Read the model definition and answer for the solid it produces. Units are mm, in the model's axes. A direction names the side the tool comes from. Coordinates: 2 decimals unless noted, no trailing zeros. Order: outer loops, then holes, each group sorted by start corner. A loop starts at its lowest first (then second) coordinate and runs counter-clockwise, first axis right, second up. Notation, with made-up numbers: M 50.5,48 L 100.5,48 A14 cw 100.5,62 Z; hole C 67,-16 d1. An arc over 180 degrees is marked long. Use a Markdown table: item, result. Add a question column.
1) The mould has two halves that part along X. Classify faces 1 (the face through (10, -50.8, 10)), 2 (the face through (130.168, -41, -22)), 3 (the face through (-87.57, -41.41, -3.07)), 4 (the face through (-144.733, -1, -2)): released by +X, released by -X, zero draft, split by the parting line, or undercut.
2) Find section C-C on z = -2. Write down the section's boundary in (x, y), plus the area to 3 significant figures.
3) Find section D-D on y = -36.5. Write down the section's boundary in (x, z) (3 decimals).
4) Each of these flat-tipped pins is pushed along its axis until it touches: pin 1 Ø8 at (y, z) = (-35.5, 50.5) entering from +X; pin 2 Ø7 at (x, y) = (104.5, -45.5) entering from -Z; pin 3 Ø12 at (x, y) = (-70, -25) entering from +Z. Where does it stop, or does it pass through?
5) Find section B-B on x = 44. Write down the section's boundary in (y, z), plus the area to 3 significant figures.
6) Find the intervals of material crossed by probe 1 along Z at (x, y) = (75, 28); probe 2 along Y at (x, z) = (-126.5, -5); probe 3 along X at (y, z) = (-43.5, 20.5), in increasing order. Write a range as [from, to].
7) Find section A-A on y = 30.5. Write down the section's boundary in (x, z).
8) For faces 5 (the face through (-5, -1, 63.942)), 6 (the face through (-107, -41, 3.617)), 7 (the face through (28.568, -1, 41)), 8 (the face through (-104, -1, 25.842)), determine the directions among +Z, -Z, +X, -X, +Y, -Y from which every point of the face is accessible in a straight line to the end or side of a thin tool.
from build123d import *

# Parameters (mm, degrees)
F1_DEPTH = 50.8
F3_DEPTH = 19.05


with BuildPart() as f1:
    # F0 (on Front) → F1 (new body, symmetric)
    with BuildSketch(Plane.XZ):
        with BuildLine():
            Line((-71.399881, 25.841707), (-138.383388, 25.841707))
            ThreePointArc((-138.383388, 25.841707), (-142.873516, 23.981835), (-144.733388, 19.491707))
            Line((-144.733388, 19.491707), (-144.733388, -24.958293))
            Line((-144.733388, -24.958293), (-119.333388, -24.958293))
            Line((-119.333388, -24.958293), (-119.333388, -18.608293))
            ThreePointArc((-119.333388, -18.608293), (-112.823836, -2.892845), (-97.108388, 3.616707))
            Line((-97.108388, 3.616707), (-90.758388, 3.616707))
            ThreePointArc((-90.758388, 3.616707), (-75.042939, -2.892845), (-68.533388, -18.608293))
            Line((-68.533388, -18.608293), (-68.533388, -24.958293))
            Line((-68.533388, -24.958293), (83.866612, -24.958293))
            Line((83.866612, -24.958293), (83.866612, -18.608293))
            ThreePointArc((83.866612, -18.608293), (90.376164, -2.892845), (106.091612, 3.616707))
            Line((106.091612, 3.616707), (112.441612, 3.616707))
            ThreePointArc((112.441612, 3.616707), (128.157061, -2.892845), (134.666612, -18.608293))
            Line((134.666612, -18.608293), (134.666612, -24.958293))
            Line((134.666612, -24.958293), (168.267654, -24.958293))
            Line((168.267654, -24.958293), (168.267654, 25.841707))
            Line((168.267654, 25.841707), (28.567654, 25.841707))
            Line((28.567654, 25.841707), (28.567654, 57.591707))
            ThreePointArc((28.567654, 57.591707), (26.707782, 62.081835), (22.217654, 63.941707))
            Line((22.217654, 63.941707), (-32.065853, 63.941707))
            ThreePointArc((-32.065853, 63.941707), (-34.678483, 63.379337), (-36.828353, 61.791837))
            Line((-36.828353, 61.791837), (-66.637381, 27.991577))
            ThreePointArc((-66.637381, 27.991577), (-68.78725, 26.404077), (-71.399881, 25.841707))
        make_face()
        with BuildLine():
            Line((-119.333388, -18.608293), (-119.333388, -24.958293))
            Line((-119.333388, -24.958293), (-68.533388, -24.958293))
            Line((-68.533388, -24.958293), (-68.533388, -18.608293))
            ThreePointArc((-68.533388, -18.608293), (-75.042939, -2.892845), (-90.758388, 3.616707))
            Line((-90.758388, 3.616707), (-97.108388, 3.616707))
            ThreePointArc((-97.108388, 3.616707), (-112.823836, -2.892845), (-119.333388, -18.608293))
        make_face()
        with BuildLine():
            Line((83.866612, -18.608293), (83.866612, -24.958293))
            Line((83.866612, -24.958293), (134.666612, -24.958293))
            Line((134.666612, -24.958293), (134.666612, -18.608293))
            ThreePointArc((134.666612, -18.608293), (128.157061, -2.892845), (112.441612, 3.616707))
            Line((112.441612, 3.616707), (106.091612, 3.616707))
            ThreePointArc((106.091612, 3.616707), (90.376164, -2.892845), (83.866612, -18.608293))
        make_face()
    extrude(amount=F1_DEPTH, both=True)

    # F2 (on face) → F3 (cut)
    with BuildSketch(Plane.XZ.offset(50.8)):
        with BuildLine():
            Line((-132.033388, -18.608293), (-132.033388, -24.958293))
            Line((-132.033388, -24.958293), (-81.233388, -24.958293))
            Line((-81.233388, -24.958293), (-81.233388, -18.608293))
            ThreePointArc((-81.233388, -18.608293), (-87.742939, -2.892845), (-103.458388, 3.616707))
            Line((-103.458388, 3.616707), (-109.808388, 3.616707))
            ThreePointArc((-109.808388, 3.616707), (-125.523836, -2.892845), (-132.033388, -18.608293))
        make_face()
        with BuildLine():
            Line((79.367654, -18.608293), (79.367654, -24.958293))
            Line((79.367654, -24.958293), (130.167654, -24.958293))
            Line((130.167654, -24.958293), (130.167654, -18.608293))
            ThreePointArc((130.167654, -18.608293), (123.658102, -2.892845), (107.942654, 3.616707))
            Line((107.942654, 3.616707), (101.592654, 3.616707))
            ThreePointArc((101.592654, 3.616707), (85.877206, -2.892845), (79.367654, -18.608293))
        make_face()
    extrude(amount=-F3_DEPTH, mode=Mode.SUBTRACT)


solid = f1.part
Check result:
| question | item | result |
|---|---|---|
| 1 | face 1 | zero draft |
| 1 | face 2 | undercut |
| 1 | face 3 | undercut |
| 1 | face 4 | released by -X |
| 2 | outline | M -144.73,-50.8 L -124.58,-50.8 L -124.58,-31.75 L -88.69,-31.75 L -88.69,-50.8 L 86.82,-50.8 L 86.82,-31.75 L 122.71,-31.75 L 122.71,-50.8 L 168.27,-50.8 L 168.27,50.8 L -144.73,50.8 Z |
| 2 | area | 30,400 mm2 |
| 3 | outline | M -144.733,-24.958 L -132.033,-24.958 L -132.033,-18.608 A22.225 cw -109.808,3.617 L -103.458,3.617 A22.225 cw -81.233,-18.608 L -81.233,-24.958 L 79.368,-24.958 L 79.368,-18.608 A22.225 cw 101.593,3.617 L 107.943,3.617 A22.225 cw 130.168,-18.608 L 130.168,-24.958 L 168.268,-24.958 L 168.268,25.842 L 28.568,25.842 L 28.568,57.592 A6.35 ccw 22.218,63.942 L -32.066,63.942 A6.35 ccw -36.828,61.792 L -66.637,27.992 A6.35 cw -71.4,25.842 L -138.383,25.842 A6.35 ccw -144.733,19.492 Z |
| 4 | pin 1 | stops at x = 28.57 |
| 4 | pin 2 | stops at z = 3.61 |
| 4 | pin 3 | stops at z = 30.98 |
| 5 | outline | M -50.8,-24.96 L 50.8,-24.96 L 50.8,25.84 L -50.8,25.84 Z |
| 5 | area | 5,160 mm2 |
| 6 | probe 1 | z = [-24.96, 25.84] |
| 6 | probe 2 | y = [-31.75, 50.8] |
| 6 | probe 3 | x = [-144.65, 168.27] |
| 7 | outline | M -144.73,-24.96 L 168.27,-24.96 L 168.27,25.84 L 28.57,25.84 L 28.57,57.59 A6.35 ccw 22.22,63.94 L -32.07,63.94 A6.35 ccw -36.83,61.79 L -66.64,27.99 A6.35 cw -71.4,25.84 L -138.38,25.84 A6.35 ccw -144.73,19.49 Z |
| 8 | face 5 | +Z, +X, -X, +Y, -Y |
| 8 | face 6 | -Z, -Y |
| 8 | face 7 | +Z, +X, +Y, -Y |
| 8 | face 8 | +Z, -X, +Y, -Y |
